Geometry: final body of the model. Coordinates: model frame, mm. A direction names the side the tool comes from. Round coordinates to 2 decimals unless told otherwise and drop trailing zeros. Order: outer loops, then holes, each group sorted by start corner. A loop starts at its lowest first (then second) coordinate and runs counter-clockwise, first axis right, second up. Notation, with made-up numbers: M 63.5,70.5 L 122.5,70.5 A24 ccw 122.5,83.5 Z; hole C 64,-7.5 d6. An arc over 180 degrees is marked long. Put each result on its own line as item: value. Start each with the question number.
1) Section D-D, the plane x = 0. Return loops of the section in (y, z).
2) Access query for faces 5 (the cylindrical face through (-1.978, 0.493, -2.579)), 6 (the cylindrical face through (-9, 1, 0)). Directions: +Z, -Z, +X, -X, +Y, -Y. A direction counts if a zero-diameter tool reaches every point of the face in a straight line with its end or side. Return the directions, or none.
3) Material intervals for probe 1 along X at (y, z) = (0.75, 0); probe 2 along X at (y, z) = (1.8, 0); probe 3 along Z at (x, y) = (-0.25, 1.35), sorted ascending. Write a range as [from, to].
4) Section C-C, the plane y = 1.5. Return loops of the section in (x, z), then the cut area to 3 significant figures.
5) First-contact query: P1, Ø1, axis at y = 2, z = -2.5, coming from the -X side. Flat tip, straight axial feed; report the tip coordinate or a pass-through.
6) Draft query along Z for faces 1 (the cylindrical face through (1, 1, -8)), 2 (the cylindrical face through (-9.76, 1.48, -2.17)), 3 (the flat face through (-4, 0, 0)), 4 (the cylindrical face through (-5.496, 1.479, 0.065)). Return one class per face: pulls with the +Z half, pulls with the -Z half, needs draft (parallel to the pull), parting line crosses it, or undercut.
7) Section B-B, the plane z = 8. Return loops of the section in (x, y).
8) Section A-A, the plane x = -8. Return loops of the section in (y, z).
from build123d import *

# Parameters (mm, degrees)
SKETCH_1_R          = 10
EXTRUDE_1_DEPTH     = 3
SKETCH_2_R          = 1
SKETCH_2_R_2        = 0.5
CUT_EXTRUDE_1_DEPTH = 3
SKETCH_4_R          = 3.25
CUT_EXTRUDE_5_DEPTH = 1
CUT_EXTRUDE_6_REACH = 16.283
SKETCH_5_R          = 2.5


with BuildPart() as part:
    # 草图1 → 凸台-拉伸1 (new body)
    with BuildSketch(Plane(origin=(0, 0, 0), x_dir=(1, 0, 0), z_dir=(0, 1, 0))):
        with Locations(Location((0, 0, 0), (0, 0, 270))):
            Circle(SKETCH_1_R)
    extrude(amount=EXTRUDE_1_DEPTH)

    # 草图2 → 切除-拉伸1 (cut)
    with BuildSketch(Plane(origin=(0, 0, 0), x_dir=(1, 0, 0), z_dir=(0, 1, 0))):
        with Locations(Location((8, 0, 0), (0, 0, 270))):
            Circle(SKETCH_2_R)
        with Locations(Location((5, 0, 0), (0, 0, 270))):
            Circle(SKETCH_2_R_2)
        with Locations(Location((-5, 0, 0), (0, 0, 90))):
            Circle(SKETCH_2_R_2)
        with Locations(Location((-8, 0, 0), (0, 0, 90))):
            Circle(SKETCH_2_R)
        with Locations(Location((0, 8, 0), (0, 0, 90))):
            Circle(SKETCH_2_R)
        with Locations(Location((0, -8, 0), (0, 0, 270))):
            Circle(SKETCH_2_R)
    extrude(amount=CUT_EXTRUDE_1_DEPTH, mode=Mode.SUBTRACT)

    # 草图4 → 切除-拉伸5 (cut)
    with BuildSketch(Plane(origin=(0, 0, 0), x_dir=(1, 0, 0), z_dir=(0, 1, 0))):
        with Locations(Location((0, 0, 0), (0, 0, 270))):
            Circle(SKETCH_4_R)
    extrude(amount=CUT_EXTRUDE_5_DEPTH, mode=Mode.SUBTRACT)

    # 草图5 → 切除-拉伸6 (cut, up to next)
    with BuildSketch(Plane.XZ.offset(-1), mode=Mode.PRIVATE) as cut_extrude_6_sk1:
        with Locations(Location((0, 0, 0), (0, 0, 270))):
            Circle(SKETCH_5_R)
    cut_extrude_6_tool1 = extrude(cut_extrude_6_sk1.sketch, amount=-CUT_EXTRUDE_6_REACH, mode=Mode.PRIVATE) & part.part
    add(cut_extrude_6_tool1.solids().sort_by_distance((0, 1, 0))[0], mode=Mode.SUBTRACT)


solid = part.part
Result sheet:
1. outline: M 0,-10 L 3,-10 L 3,-9 L 0,-9 Z; M 0,-7 L 3,-7 L 3,-2.5 L 1,-2.5 L 1,-3.25 L 0,-3.25 Z; M 0,3.25 L 1,3.25 L 1,2.5 L 3,2.5 L 3,7 L 0,7 Z; M 0,9 L 3,9 L 3,10 L 0,10 Z
2. face 5: -Y
2. face 6: +Y, -Y
3. probe 1: x = [-10, -9], [-7, -5.5], [-4.5, -3.25], [3.25, 4.5], [5.5, 7], [9, 10]
3. probe 2: x = [-10, -9], [-7, -5.5], [-4.5, -2.5], [2.5, 4.5], [5.5, 7], [9, 10]
3. probe 3: z = [-10, -8.97], [-7.03, -2.49], [2.49, 7.03], [8.97, 10]
4. outline: C 0,0 d20; hole C -8,0 d2; hole C -5,0 d1; hole C 0,0 d5; hole C 0,-8 d2; hole C 0,8 d2; hole C 5,0 d1; hole C 8,0 d2
4. area: 280 mm2
5. P1: stops at x = -9.8
6. face 1: undercut
6. face 2: parting line crosses it
6. face 3: needs draft
6. face 4: undercut
7. outline: M -6,0 L -1,0 L -1,3 L -6,3 Z; M 1,0 L 6,0 L 6,3 L 1,3 Z
8. outline: M 0,-6 L 3,-6 L 3,-1 L 0,-1 Z; M 0,1 L 3,1 L 3,6 L 0,6 Z
